Geometry: see drawing. Coordinates: mm, zero at the bounding-box minimum. A direction names the side the tool comes from. Give positions to 0.01 mm unless a question says otherwise; leave off trailing zeros. Write each loop counter-clockwise with the first axis right and the second up, starting at its lowest first coordinate (ties: lowest second). Pieces come first, ordered by that corner, then holes. Notation, with made-up numbers: M 16.25,44.25 L 75.25,44.25 A17 ccw 75.25,56.25 Z; hole C 71,40.5 d10. An arc over 180 degrees is marked long. Use a Markdown table: item, result. Add a question column.
(1) Pin query (flat end, axial travel): pin 1 Ø3 at (x, y) = (8, 5) entering from +Z; pin 2 Ø2 at (x, y) = (13.5, 3.5) entering from -Z; pin 3 Ø5.5 at (x, z) = (6.75, 8) entering from +Y; pin 4 Ø1.5 at (y, z) = (7, 4) entering from +X. Return the tip coordinate at first contact, or that it passes through.
(2) Reachability of the marked faces 1, 2 and 3 from +Z, -Z, +X, -X, +Y, -Y: full face, straight path, thin tool, end or side. Return the list, or none.
(3) Material intervals for L1, parallel to X at y = 6.75, z = 8.25; L2, parallel to X at y = 1.25, z = 11.75 (1 decimal); L3, parallel to Y at x = 20, z = 10, sorted ascending.
(4) Cut plane C-C (y = 8.5). Output: boundary loops of the cut face in (x, z).
(5) Cut plane B-B (x = 9). Output: boundary loops of the cut face in (y, z).
(6) Cut plane A-A (z = 10). Output: boundary loops of the cut face in (x, y), plus the area to 3 significant figures.
(7) Cut plane D-D (x = 22.5). Output: boundary loops of the cut face in (y, z), plus the area to 3 significant figures.
(8) Draft query along X for the marked faces 4, 5 and 6. Return one class per face: released by +X, released by -X, zero draft, split by the parting line, or undercut.
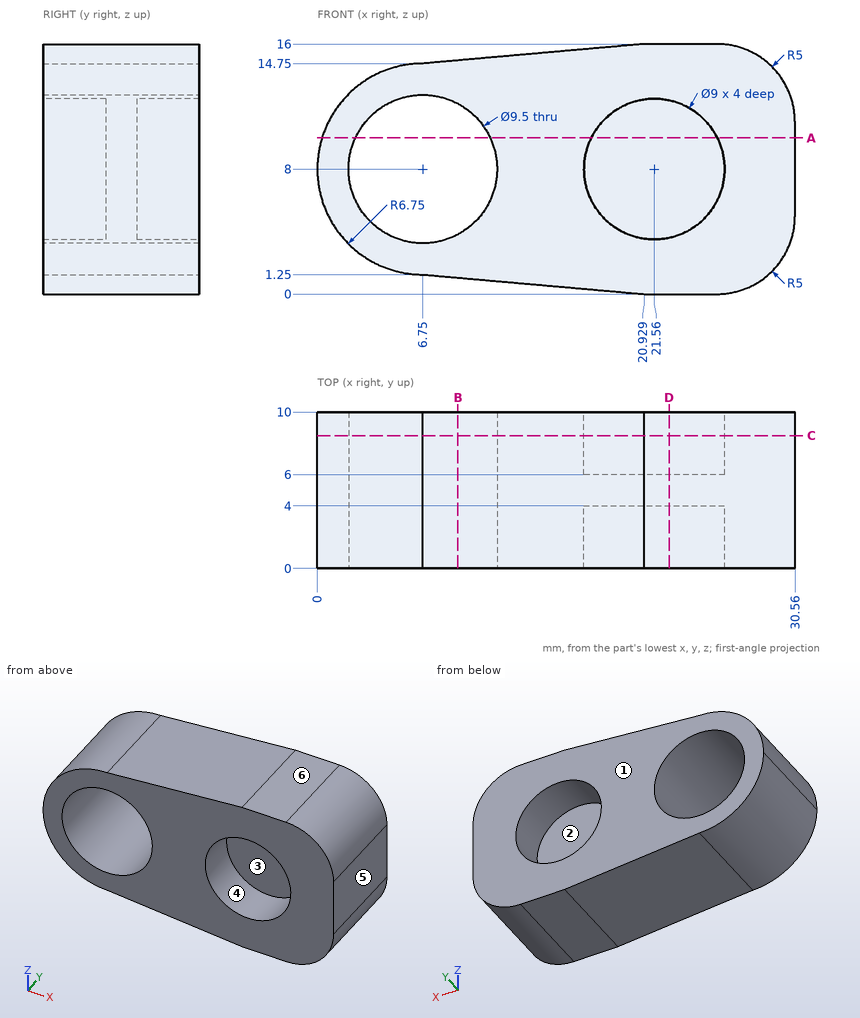
Answer list:
| question | item | result |
|---|---|---|
| 1 | pin 1 | z = 14.99 |
| 1 | pin 2 | z = 0.57 |
| 1 | pin 3 | through |
| 1 | pin 4 | x = 30.55 |
| 2 | face 1 | +Z, -Z, +X, -X, +Y |
| 2 | face 2 | +Y |
| 2 | face 3 | -Y |
| 3 | L1 | 0 to 2.01, 11.49 to 17.07, 26.05 to 30.56 |
| 3 | L2 | 1.1 to 3.8, 9.7 to 19.1, 24 to 30.5 |
| 3 | L3 | 4 to 6 |
| 4 | outline | M 0,8 A6.75 ccw 6.75,1.25 L 20.93,0 L 25.56,0 A5 ccw 30.56,5 L 30.56,11 A5 ccw 25.56,16 L 20.93,16 L 6.75,14.75 A6.75 ccw Z; hole C 6.75,8 d9.5; hole C 21.56,8 d9 |
| 5 | outline | M 0,1.05 L 10,1.05 L 10,3.82 L 0,3.82 Z; M 0,12.18 L 10,12.18 L 10,14.95 L 0,14.95 Z |
| 6 | outline | M 0.3,0 L 2.44,0 L 2.44,10 L 0.3,10 Z; M 11.06,0 L 17.53,0 L 17.53,4 L 25.59,4 L 25.59,0 L 30.56,0 L 30.56,10 L 25.59,10 L 25.59,6 L 17.53,6 L 17.53,10 L 11.06,10 Z |
| 6 | area | 152 mm² |
| 7 | outline | M 0,0 L 10,0 L 10,3.6 L 6,3.6 L 6,12.4 L 10,12.4 L 10,16 L 0,16 L 0,12.4 L 4,12.4 L 4,3.6 L 0,3.6 Z |
| 7 | area | 89.6 mm² |
| 8 | face 4 | undercut |
| 8 | face 5 | released by +X |
| 8 | face 6 | zero draft |
